from build123d import *

# Parameters (mm, degrees)
SKETCH1_W           = 50
SKETCH1_H           = 70
BOSS_EXTRUDE1_DEPTH = 1.6
FILLET2_R           = 5
SKETCH2_R           = 1.6
CUT_EXTRUDE1_DEPTH  = 1.6
SKETCH3_R           = 0.5
CUT_EXTRUDE2_DEPTH  = 1.6


with BuildPart() as part:
    # Sketch1 → Boss-Extrude1 (new body)
    with BuildSketch(Plane(origin=(0, 0, 0), x_dir=(1, 0, 0), z_dir=(0, 1, 0))):
        Rectangle(SKETCH1_W, SKETCH1_H)
    extrude(amount=BOSS_EXTRUDE1_DEPTH)

    # Fillet2
    fillet2_edges = [part.edges().sort_by_distance(p)[0] for p in [
        (25, 0.8, 35),
        (-25, 0.8, 35),
        (-25, 0.8, -35),
        (25, 0.8, -35),
    ]]
    fillet(fillet2_edges, radius=FILLET2_R)

    # Sketch2 → Cut-Extrude1 (cut)
    with BuildSketch(Plane(origin=(0, 1.6, 0), x_dir=(1, 0, 0), z_dir=(0, 1, 0))):
        with Locations((-20, 30)):
            Circle(SKETCH2_R)
        with Locations((20, 30)):
            Circle(SKETCH2_R)
        with Locations((20, -30)):
            Circle(SKETCH2_R)
        with Locations((-20, -30)):
            Circle(SKETCH2_R)
    extrude(amount=-CUT_EXTRUDE1_DEPTH, mode=Mode.SUBTRACT)

    # Sketch3 → Cut-Extrude2 (cut)
    with BuildSketch(Plane(origin=(0, 1.6, 0), x_dir=(1, 0, 0), z_dir=(0, 1, 0))):
        with Locations((-3.81, 25.8)):
            Circle(SKETCH3_R)
        with Locations((-1.27, 25.8)):
            Circle(SKETCH3_R)
        with Locations((1.27, 25.8)):
            Circle(SKETCH3_R)
        with Locations((3.81, 25.8)):
            Circle(SKETCH3_R)
        with Locations((-11.75, 25.8)):
            Circle(SKETCH3_R)
        with Locations((-9.21, 25.8)):
            Circle(SKETCH3_R)
        with Locations((-15.76, -20.1)):
            Circle(SKETCH3_R)
        with Locations((-13.22, -20.1)):
            Circle(SKETCH3_R)
        with Locations((-10.68, -20.1)):
            Circle(SKETCH3_R)
        with Locations((-8.14, -20.1)):
            Circle(SKETCH3_R)
        with Locations((-5.6, -20.1)):
            Circle(SKETCH3_R)
        with Locations((-3.06, -20.1)):
            Circle(SKETCH3_R)
        with Locations((-0.52, -20.1)):
            Circle(SKETCH3_R)
        with Locations((2.02, -20.1)):
            Circle(SKETCH3_R)
        with Locations((4.56, -20.1)):
            Circle(SKETCH3_R)
        with Locations((7.1, -20.1)):
            Circle(SKETCH3_R)
        with Locations((9.64, -20.1)):
            Circle(SKETCH3_R)
        with Locations((12.18, -20.1)):
            Circle(SKETCH3_R)
        with Locations((14.72, -20.1)):
            Circle(SKETCH3_R)
        with Locations((17.26, -20.1)):
            Circle(SKETCH3_R)
        with Locations((19.8, -20.1)):
            Circle(SKETCH3_R)
        with Locations((-15.76, -4.86)):
            Circle(SKETCH3_R)
        with Locations((-13.22, -4.86)):
            Circle(SKETCH3_R)
        with Locations((-10.68, -4.86)):
            Circle(SKETCH3_R)
        with Locations((-8.14, -4.86)):
            Circle(SKETCH3_R)
        with Locations((-5.6, -4.86)):
            Circle(SKETCH3_R)
        with Locations((-3.06, -4.86)):
            Circle(SKETCH3_R)
        with Locations((-0.52, -4.86)):
            Circle(SKETCH3_R)
        with Locations((2.02, -4.86)):
            Circle(SKETCH3_R)
        with Locations((4.56, -4.86)):
            Circle(SKETCH3_R)
        with Locations((7.1, -4.86)):
            Circle(SKETCH3_R)
        with Locations((9.64, -4.86)):
            Circle(SKETCH3_R)
        with Locations((12.18, -4.86)):
            Circle(SKETCH3_R)
        with Locations((14.72, -4.86)):
            Circle(SKETCH3_R)
        with Locations((17.26, -4.86)):
            Circle(SKETCH3_R)
        with Locations((19.8, -4.86)):
            Circle(SKETCH3_R)
        with Locations((-3.35, 1.86)):
            Circle(SKETCH3_R)
        with Locations((-0.81, 1.86)):
            Circle(SKETCH3_R)
        with Locations((1.73, 1.86)):
            Circle(SKETCH3_R)
        with Locations((4.27, 1.86)):
            Circle(SKETCH3_R)
        with Locations((6.81, 1.86)):
            Circle(SKETCH3_R)
        with Locations((9.35, 1.86)):
            Circle(SKETCH3_R)
        with Locations((-3.35, 17.1)):
            Circle(SKETCH3_R)
        with Locations((-0.81, 17.1)):
            Circle(SKETCH3_R)
        with Locations((1.73, 17.1)):
            Circle(SKETCH3_R)
        with Locations((4.27, 17.1)):
            Circle(SKETCH3_R)
        with Locations((6.81, 17.1)):
            Circle(SKETCH3_R)
        with Locations((9.35, 17.1)):
            Circle(SKETCH3_R)
        with Locations((-12.7, -28.5)):
            Circle(SKETCH3_R)
        with Locations((-10.16, -28.5)):
            Circle(SKETCH3_R)
        with Locations((-7.62, -28.5)):
            Circle(SKETCH3_R)
        with Locations((-5.08, -28.5)):
            Circle(SKETCH3_R)
        with Locations((-2.54, -28.5)):
            Circle(SKETCH3_R)
        with Locations((0, -28.5)):
            Circle(SKETCH3_R)
        with Locations((2.54, -28.5)):
            Circle(SKETCH3_R)
        with Locations((5.08, -28.5)):
            Circle(SKETCH3_R)
        with Locations((7.62, -28.5)):
            Circle(SKETCH3_R)
        with Locations((10.16, -28.5)):
            Circle(SKETCH3_R)
        with Locations((12.7, -28.5)):
            Circle(SKETCH3_R)
        with Locations((17, 15.85)):
            Circle(SKETCH3_R)
        with Locations((17, 13.31)):
            Circle(SKETCH3_R)
        with Locations((17, 10.77)):
            Circle(SKETCH3_R)
        with Locations((17, 3.15)):
            Circle(SKETCH3_R)
        with Locations((17, 5.69)):
            Circle(SKETCH3_R)
        with Locations((17, 8.23)):
            Circle(SKETCH3_R)
        with Locations((-18.5, 20.6)):
            Circle(SKETCH3_R)
        with Locations((-18.5, 18.06)):
            Circle(SKETCH3_R)
        with Locations((-18.5, 11.86)):
            Circle(SKETCH3_R)
        with Locations((-18.5, 9.32)):
            Circle(SKETCH3_R)
        with Locations((-16, 5.6)):
            Circle(SKETCH3_R)
        with Locations((-16, -0.9)):
            Circle(SKETCH3_R)
        with Locations((-20.5, -0.9)):
            Circle(SKETCH3_R)
        with Locations((-20.5, 5.6)):
            Circle(SKETCH3_R)
        with Locations((9.5, 26.5)):
            Circle(SKETCH3_R)
        with Locations((16.571067812, 19.428932188)):
            Circle(SKETCH3_R)
        with Locations((-6.928932188, 10.928932188)):
            Circle(SKETCH3_R)
        with Locations((-14, 18)):
            Circle(SKETCH3_R)
        with Locations((-14, 9.5)):
            Circle(SKETCH3_R)
        with Locations((-6.928932188, 2.428932188)):
            Circle(SKETCH3_R)
    extrude(amount=-CUT_EXTRUDE2_DEPTH, mode=Mode.SUBTRACT)


solid = part.part
For this review, take the finished solid that the model builds, in its own axes (mm). Give positions to 0.01 mm unless a question says otherwise; leave off trailing zeros. Answer as a JSON object with one key per item and string values. Group by question number.
Item 1: Wall thickness on line 1 along Z through (x, y) = (20, 0.95); line 2 along X through (y, z) = (0.15, -10.5); line 3 along Z through (x, y) = (-19.5, 0.95): over which ranges is each line inside the solid? List them lowest first.
Item 2: Take a section at A-A on y = 0.4. Give the number of separate pieces and of enclosed holes in the cut face, and give its area (3 significant figures).
Item 3: Clearance check with flat-ended pins moving along their axes: pin 1 Ø3.5 at (x, z) = (20, 30) entering from +Y; pin 2 Ø2.5 at (x, z) = (20, -30) entering from -Y. State where each tip first meets the part, or that it passes through.
Item 4: Draft analysis for pull direction X (two halves, no side actions). For faces 1 (the cylindrical face through (18.82, 0.81, 28.92)), 2 (the cylindrical face through (-20.208, 0.811, 28.414)), 3 (the flat face through (-25, 1, 0)), 4 (the flat face through (0, 0, 0)), state which applies: pulls with the +X half, pulls with the -X half, needs draft (parallel to the pull), parting line crosses it, or undercut.
Reported:
{
 "1": {"line 1": "-35 to -31.6, -28.4 to 4.4, 5.32 to 19.64, 20.56 to 28.4, 31.6 to 35", "line 2": "-25 to -7.19, -6.67 to 16.58, 17.42 to 25", "line 3": "-35 to -31.52, -28.48 to 28.48, 31.52 to 35"},
 "2": {"separate pieces": "1", "enclosed holes": "83", "area": "3,380 mm^2"},
 "3": {"pin 1": "y = 1.6", "pin 2": "through"},
 "4": {"face 1": "undercut", "face 2": "undercut", "face 3": "pulls with the -X half", "face 4": "needs draft"}
}
